Work out the finished part from the listing and answer in its coordinate system (mm). A direction names the side the tool comes from. Give positions to 0.01 mm unless a question says otherwise; leave off trailing zeros. Loops run counter-clockwise (first coordinate to the right, second up) from the corner with the lowest first, then second, coordinate; pieces in that order, holes last. Notation, with made-up numbers: (-15.75, -15.5) - (40.25, -15.5) arc R8 cw to (40.25, -11.5) - close; hole circle Ø1 at (7.5, -34.5). An arc over 180 degrees is marked (long way). One line per item, written item: value.
from build123d import *

# Parameters (mm, degrees)
SKETCH1_R           = 1.25
BOSS_EXTRUDE1_DEPTH = 6
SKETCH2_R           = 2.1
CUT_EXTRUDE1_DEPTH  = 3


with BuildPart() as part:
    # Sketch1 → Boss-Extrude1 (new body)
    with BuildSketch(Plane.XY):
        Polygon((-41.523066959, 14), (-41.523066959, -14), (6.974355653, -28), (31.223066959, -14), (31.223066959, 14), (6.974355653, 28), align=None)
        with Locations((-5.15, 0)):
            Circle(SKETCH1_R, mode=Mode.SUBTRACT)
    extrude(amount=BOSS_EXTRUDE1_DEPTH)

    # Sketch2 → Cut-Extrude1 (cut)
    with BuildSketch(Plane(origin=(0, 0, 0), x_dir=(-1, 0, 0), z_dir=(0, 0, -1))):
        with Locations((5.15, 0)):
            Circle(SKETCH2_R)
    extrude(amount=-CUT_EXTRUDE1_DEPTH, mode=Mode.SUBTRACT)


solid = part.part
1. For faces 4 (the cylindrical face through (-3.05, 0.09, 1.48)), 5 (the flat face through (-6, 7, 6)), determine the directions among +Z, -Z, +X, -X, +Y, -Y from which every point of the face is accessible in a straight line to the end or side of a thin tool.
Output:
face 4: -Z
face 5: +Z, +X, -X, +Y, -Y
2. Section C-C (y = 0) is taken. Write down the section's boundary in (x, z).
Output:
outline: (-41.52, 0) - (-7.25, 0) - (-7.25, 3) - (-6.4, 3) - (-6.4, 6) - (-41.52, 6) - close; (-3.9, 3) - (-3.05, 3) - (-3.05, 0) - (31.22, 0) - (31.22, 6) - (-3.9, 6) - close
3. Section A-A (x = -5.15) is taken. Write down the section's boundary in (y, z).
Output:
outline: (-24.5, 0) - (-2.1, 0) - (-2.1, 3) - (-1.25, 3) - (-1.25, 6) - (-24.5, 6) - close; (1.25, 3) - (2.1, 3) - (2.1, 0) - (24.5, 0) - (24.5, 6) - (1.25, 6) - close
4. Flat-ended cylindrical pins translate along their axes: pin 1 Ø4 at (x, y) = (-5.15, 0) entering from -Z; pin 2 Ø3 at (x, z) = (-25, 5) entering from +Y; pin 3 Ø2 at (x, y) = (-5.15, 0) entering from -Z. Find the tip coordinate at first contact, or state that the pin passes through.
Output:
pin 1: stops at z = 3
pin 2: stops at y = 19.2
pin 3: passes through
5. Section B-B (z = 3.8) is taken. Write down the section's boundary in (x, y), and give its area (3 significant figures).
Output:
outline: (-41.52, -14) - (6.97, -28) - (31.22, -14) - (31.22, 14) - (6.97, 28) - (-41.52, 14) - close; hole circle Ø2.5 at (-5.15, 0)
area: 3,050 mm²
6. Find the intervals of material crossed by line 1 along X through (y, z) = (0, 4.4); line 2 along Y through (x, z) = (7, 1.65); line 3 along Y through (x, z) = (-4.5, 1.5), in increasing order.
Output:
line 1: x = -41.52 to -6.4, -3.9 to 31.22
line 2: y = -27.99 to 27.99
line 3: y = -24.69 to -2, 2 to 24.69
7. Section D-D (y = -23.5) is taken. Write down the section's boundary in (x, z).
Output:
outline: (-8.61, 0) - (14.77, 0) - (14.77, 6) - (-8.61, 6) - close
8. The mould has two halves that part along X. Classify faces 1 (the flat face through (31.223, 0, 3)), 2 (the flat face through (-7, 0, 3)), 3 (the flat face through (-6, 7, 0)): released by +X, released by -X, zero draft, split by the parting line, or undercut.
Output:
face 1: released by +X
face 2: undercut
face 3: zero draft
